Here's how the part is built. I have some questions about the finished solid (model axes, mm). A direction names the side the tool comes from. Round coordinates to 2 decimals unless told otherwise and drop trailing zeros. Loops run counter-clockwise (first coordinate to the right, second up) from the corner with the lowest first, then second, coordinate; pieces in that order, holes last. Notation, with made-up numbers: (11.25, 39.25) - (21.25, 39.25) arc R20 cw to (21.25, 56.25) - close; hole circle Ø6 at (20, 45.5). An arc over 180 degrees is marked (long way). Answer as a JSON object with one key per item and string values. Group by question number.
1) If I drill on line 1 along Y through (x, z) = (7, 8); line 2 along Z through (x, y) = (11.5, 11); line 3 along X through (y, z) = (14.5, 7.75), over which ranges is the centre line in solid material (lowest first)? Write a range as [from, to].
2) I want a section at A-A, the plane x = 12. Please give me the cut outline in (y, z), then the cut area to 3 significant figures.
3) Will these pins go through, and if not, where does the flat tip stop? P1, Ø12, axis at x = -5.5, z = -7, coming from the -Y side; P2, Ø5, axis at x = 10, z = 2.5, coming from the +Y side.
4) Which directions (+Z, -Z, +X, -X, +Y, -Y) give clear straight access to the entire face, cutting with the end or side of a thin tool? Please do faces 1 (the face through (-4, 8, 10)), 2 (the face through (9, 14, -5)).
5) I want a section at B-B, the plane y = 12.5. Please give me the cut outline in (x, z).
6) I want a section at C-C, the plane x = -2.75. Please give me the cut outline in (y, z) (3 decimals), then the cut area to 3 significant figures.
from build123d import *

# Parameters (mm, degrees)
SKETCH_1_W          = 30
SKETCH_1_H          = 20
EXTRUDE_1_DEPTH     = 20
CUT_EXTRUDE_3_REACH = 39.417
SKETCH_5_W          = 15
SKETCH_5_H          = 15


with BuildPart() as part:
    # 草圖1 → 填料-伸長1 (new body)
    with BuildSketch(Plane(origin=(0, 0, 0), x_dir=(1, 0, 0), z_dir=(0, 1, 0))):
        Rectangle(SKETCH_1_W, SKETCH_1_H)
    extrude(amount=EXTRUDE_1_DEPTH)

    # 除料-伸長3: up to this plane
    cut_extrude_3_end = Plane(origin=(7.5, 5, 2.5), z_dir=(-0.8017837257372732, -0.5345224838248487, -0.2672612419124243))
    # 草圖5 → 除料-伸長3 (cut, up to the surface)
    with BuildSketch(Plane(origin=(15, 0, 0), x_dir=(0, 0, -1), z_dir=(1, 0, 0)), mode=Mode.PRIVATE) as cut_extrude_3_sk1:
        with Locations((-2.5, 12.5)):
            Rectangle(SKETCH_5_W, SKETCH_5_H)
    cut_extrude_3_tool1 = split(extrude(cut_extrude_3_sk1.sketch, amount=-CUT_EXTRUDE_3_REACH, mode=Mode.PRIVATE), bisect_by=cut_extrude_3_end, keep=Keep.BOTH, mode=Mode.PRIVATE)
    add(cut_extrude_3_tool1.solids().sort_by_distance((15, 12.5, 2.5))[0], mode=Mode.SUBTRACT)


solid = part.part
Outcome:
{
 "1": {"line 1": "[0, 5]", "line 2": "[-10, -5]", "line 3": "[-15, -0.58]"},
 "2": {"outline": "(0, -10) - (20, -10) - (20, -5) - (5, -5) - (5, 10) - (0, 10) - close", "area": "175 mm^2"},
 "3": {"P1": "y = 0", "P2": "y = 5.2"},
 "4": {"face 1": "+Z, +X, -X, +Y, -Y", "face 2": "+Z, +X, +Y"},
 "5": {"outline": "(-15, -10) - (15, -10) - (15, -5) - (5, -5) - (0, 10) - (-15, 10) - close"},
 "6": {"outline": "(0, -10) - (20, -10) - (20, 3.25) - (16.625, 10) - (0, 10) - close", "area": "389 mm^2"}
}
